Autodesk Fusion 360 part; units mm, degrees
sketch "Esquisse1" plane through (0, 0, 0) normal (0, 0, 1) x (1, 0, 0)
  circle A0 centre (47.4696, 29.6196) radius 5.5
  circle A1 centre (47.4696, 29.6196) radius 3.5
  line L0 (47.4696, 29.6196) -> (47.4696, 24.1196)
  line L1 (46.4696, 26.2655) -> (48.4696, 26.2655)
  line L2 (48.4696, 26.2655) -> (48.4696, 24.1196)
  line L3 (48.4696, 24.1196) -> (46.4696, 24.1196)
  line L4 (46.4696, 24.1196) -> (46.4696, 26.2655)
  dimension "d5" = 7
  dimension "d6" = 2
  dimension "d7" = 1
extrude "Extrusion1" add sketch "Esquisse1" along normal blind 4 contours A0 A1 L2 L4
extrude "Extrusion2" add sketch "Esquisse1" along normal blind 1 contours A0 A1 L0 L4 | A0 L3 L4 | A0 L2 L3 | A0 A1 L0 L2
sketch "Esquisse2" plane through (0, 24.1196, 0) normal (0, -1, 0) x (1, 0, 0)
  line L0 (46.4696, 0) -> (48.4696, 0)
  line L1 (48.4696, 0) -> (48.4696, 1)
  line L2 (48.4696, 1) -> (46.4696, 1)
  line L3 (46.4696, 1) -> (46.4696, 0)
  circle A0 centre (47.4696, -9) radius 8
  circle A1 centre (47.4696, -9) radius 9
  line L4 (47.4696, 0) -> (47.4696, -9)
  line L5 (48.4696, 0) -> (46.4696, 0)
  line L6 (43.3465, -1) -> (51.5927, -1)
  line L7 (51.5927, -1) -> (52.9696, 0)
  line L8 (41.9696, 0) -> (43.3465, -1)
  line L9 (47.4696, 0) -> (41.9696, 0)
  line L10 (47.4696, 0) -> (52.9696, 0)
  line L11 (38.9843, -6) -> (55.9549, -6)
  line L12 (41.9696, -1.8761) -> (52.9696, -1.8761)
  dimension "d12" = 1
  dimension "d13" = 16
  dimension "d14" = 5.5
  dimension "d15" = 5.5
  dimension "d16" = 5
extrude "Extrusion3" add sketch "Esquisse2" against normal blind 11 contours L0 A1 L5 L8 L9 | L0 A1 L5 L7 L10 | A1 L4 L6 | A1 L4 L6 | A0 A1 L6 L12 | A0 A1 L6 L12
CAD build for the part. Positions are in the model's coordinates, mm. A direction names the side the tool comes from. Coordinates: 2 decimals unless noted, no trailing zeros. Order: outer loops, then holes, each group sorted by start corner. A loop starts at its lowest first (then second) coordinate and runs counter-clockwise, first axis right, second up. Notation, with made-up numbers: M -4.5,-8.5 L 52.5,-8.5 A9 ccw 52.5,-1.5 Z; hole C 55.5,48.25 d11. An arc over 180 degrees is marked long. Write each question's results on one line, items separated by ' | '. Start each with the question number.
Q1. Cut at B-B (x = 51.75). List the corners of the cut face in (y, z).
Q2. Pull direction X, two halves, no side cores. Call faces 4 (the cylindrical face through (47.242, 35.115, 1.972)), 5 (the flat face through (48.47, 25, 2)), 6 (the flat face through (42.648, 29.543, -0.493)), 7 (the flat face through (43, 25, 0)): +X half, -X half, draft (parallel to the pull), parting line (faces both ways), or undercut.
Q3. Drill centre lines: probe 1 along Y at (x, z) = (44.75, 3.5); probe 2 along Z at (x, y) = (51.75, 25); probe 3 along X at (y, z) = (26, 1.05). Where is each one in solid material? Low to high. Write a range as from..to.
Q4. Cut at C-C (y = 25). List the corners of the cut face in (x, z).
Q5. Cut at A-A (z = 0.85). List the corners of the cut face in (x, y), then the cut area to 3 significant figures.
Q6. Which spindle directions (+Z, -Z, +X, -X, +Y, -Y) get a long thin tool onto all of the face, cutting with end or side? Do faces 1 (the flat face through (43, 34, 0)), 2 (the flat face through (52.27, 29.54, -0.51)), 3 (the flat face through (46.47, 25, 2)). Say none if no direction does.
Q7. Cut at D-D (x = 50.5). List the corners of the cut face in (y, z).
Q8. Flat gauge pins, fed straight in: P1, Ø1, axis at x = 46.5, z = 2, coming from the +Y side; P2, Ø2.5, axis at y = 25.5, z = 2.5, coming from the -X side; P3, Ø1.5, axis at y = 29, z = 1, coming from the -X side; P4, Ø1, axis at y = 25, z = 2.5, coming from the +X side. Where does each tip first touch, or does it go through?
Found:
1) outline: M 24.12,-1.88 L 35.12,-1.88 L 35.12,-1.08 L 24.12,-1.08 Z; M 24.12,-0.89 L 35.12,-0.89 L 35.12,0 L 33.07,0 L 33.07,4 L 26.17,4 L 26.17,0 L 24.12,0 Z
2) face 4: parting line | face 5: undercut | face 6: -X half | face 7: draft
3) probe 1: 24.84..27.42, 31.82..34.4 | probe 2: -1.88..-1.08, -0.89..0 | probe 3: 43.33..46.47, 48.47..51.61
4) outline: M 41.97,-1.88 L 43.83,-1.88 A8 cw 51.11,-1.88 L 52.97,-1.88 A9 ccw 51.59,-1 L 52.97,0 L 50.45,0 L 50.45,4 L 48.47,4 L 48.47,1 L 46.47,1 L 46.47,4 L 44.48,4 L 44.48,0 L 41.97,0 L 43.35,-1 A9 ccw Z
5) outline: M 46.47,24.12 L 48.47,24.12 L 48.47,24.21 A5.5 ccw long 46.47,24.21 Z; hole C 47.47,29.62 d7 | area: 56.6 mm²
6) face 1: +Z, -X, +Y | face 2: +X, +Y, -Y | face 3: +Z, -Y
7) outline: M 24.12,-1.6 L 35.12,-1.6 L 35.12,0 L 34.21,0 L 34.21,4 L 31.37,4 L 31.37,0 L 27.87,0 L 27.87,4 L 25.03,4 L 25.03,0 L 24.12,0 Z
8) P1: y = 35.1 | P2: x = 42.78 | P3: x = 41.97 | P4: x = 51.11
